Geometry check sheet. Reference: the model listing, model coordinates, mm. A direction names the side the tool comes from. Coordinates: 2 decimals unless noted, no trailing zeros. Write each loop counter-clockwise with the first axis right and the second up, starting at its lowest first coordinate (ties: lowest second). Pieces come first, ordered by that corner, then holes. Notation, with made-up numbers: (17, 82) - (57, 82) arc R24 cw to (57, 114) - close; hole circle Ø5 at (6.25, 82). An arc over 180 degrees is marked (long way). Answer as a JSON object with one key per item and string values. Group by question number.
from build123d import *

# Parameters (mm, degrees)
BOSS_EXTRUDE1_DEPTH      = 25.4
BOSS_EXTRUDE1_DEPTH_BACK = 12.7
SKETCH1_W                = 210.82
SKETCH1_H                = 6.35
SKETCH1_3_W              = 210.82
SKETCH1_3_H              = 90.17
SKETCH1_3_R              = 14.2875
BOSS_EXTRUDE2_DEPTH      = 12.7


with BuildPart() as part:
    # Sketch1 → Boss-Extrude1 (new, two sides: drawn at the far end of the back side and taken through both)
    with BuildSketch(Plane.XY.offset(-BOSS_EXTRUDE1_DEPTH_BACK)):
        with Locations((0, 48.26)):
            Rectangle(SKETCH1_W, SKETCH1_H)
        Polygon((-105.41, 51.435), (-111.76, 51.435), (-111.76, -51.435), (-105.41, -51.435), (-105.41, -45.085), (-105.41, 45.085), align=None)
        with Locations((0, -48.26)):
            Rectangle(SKETCH1_W, SKETCH1_H)
        Polygon((105.41, 51.435), (111.76, 51.435), (111.76, -51.435), (105.41, -51.435), (105.41, -45.085), (105.41, 45.085), align=None)
    extrude(amount=BOSS_EXTRUDE1_DEPTH + BOSS_EXTRUDE1_DEPTH_BACK)

    # Sketch1_3 → Boss-Extrude2 (add)
    with BuildSketch(Plane.XY):
        Rectangle(SKETCH1_3_W, SKETCH1_3_H)
        with Locations((25.4, 0)):
            Circle(SKETCH1_3_R, mode=Mode.SUBTRACT)
        with Locations((-25.4, 0)):
            Circle(SKETCH1_3_R, mode=Mode.SUBTRACT)
    extrude(amount=-BOSS_EXTRUDE2_DEPTH)


solid = part.part
(1) Set-up check for faces 5 (the face through (-8.8, -45.5, 25.4)), 6 (the face through (-1, 1, 0)): record each of +Z, -Z, +X, -X, +Y, -Y from which the full face is reachable in a straight line by a thin tool's end or side.
(2) Section check A-A (y = 0). Record the cut outline in (x, z).
(3) Draft check along Y on faces 1 (the face through (105.41, -1, 13)), 2 (the face through (-105.41, -1, 13)), 3 (the face through (-2, -51.435, 6)), 4 (the face through (-2, 1, -12.7)). Enter one of: +Y half, -Y half, draft (parallel to the pull), parting line (faces both ways), or undercut.
(4) Gauge pin test, flat end, axial feed: pin 1 (5 mm diameter, centred on x = 59, y = 37, fed in from +Z). Record the tip position at first contact, or that the pin passes through.
(5) Section check D-D (x = 93.5). Record the cut outline in (y, z) (3 decimals), and give its area (3 significant figures).
(6) Material ranges on L1, parallel to X at y = 11.5, z = 15; L2, parallel to Y at x = -25, z = -7 (3 decimals); L3, parallel to Y at x = 65.5, z = 16.5 (3 decimals), recorded low to high. Write a range as [from, to].
(7) Section check B-B (z = 4). Record the cut outline in (x, y) (3 decimals).
(8) Section check C-C (x = -25.4). Record the cut outline in (y, z) (1 decimal).
Conclusion:
{
 "1": {"face 5": "+Z, +X, -X, +Y, -Y", "face 6": "+Z"},
 "2": {"outline": "(-111.76, -12.7) - (-39.69, -12.7) - (-39.69, 0) - (-105.41, 0) - (-105.41, 25.4) - (-111.76, 25.4) - close; (-11.11, -12.7) - (11.11, -12.7) - (11.11, 0) - (-11.11, 0) - close; (39.69, -12.7) - (111.76, -12.7) - (111.76, 25.4) - (105.41, 25.4) - (105.41, 0) - (39.69, 0) - close"},
 "3": {"face 1": "undercut", "face 2": "undercut", "face 3": "-Y half", "face 4": "draft"},
 "4": {"pin 1": "stops at z = 0"},
 "5": {"outline": "(-51.435, -12.7) - (51.435, -12.7) - (51.435, 25.4) - (45.085, 25.4) - (45.085, 0) - (-45.085, 0) - (-45.085, 25.4) - (-51.435, 25.4) - close", "area": "1,630 mm^2"},
 "6": {"L1": "x = [-111.76, -105.41], [105.41, 111.76]", "L2": "y = [-51.435, -14.282], [14.282, 51.435]", "L3": "y = [-51.435, -45.085], [45.085, 51.435]"},
 "7": {"outline": "(-111.76, -51.435) - (111.76, -51.435) - (111.76, 51.435) - (-111.76, 51.435) - close; hole (-105.41, -45.085) - (105.41, -45.085) - (105.41, 45.085) - (-105.41, 45.085) - close"},
 "8": {"outline": "(-51.4, -12.7) - (-14.3, -12.7) - (-14.3, 0) - (-45.1, 0) - (-45.1, 25.4) - (-51.4, 25.4) - close; (14.3, -12.7) - (51.4, -12.7) - (51.4, 25.4) - (45.1, 25.4) - (45.1, 0) - (14.3, 0) - close"}
}
